Verification items for the finished model (mm, model axes). A direction names the side the tool comes from. Round coordinates to 2 decimals unless told otherwise and drop trailing zeros. Order: outer loops, then holes, each group sorted by start corner. A loop starts at its lowest first (then second) coordinate and runs counter-clockwise, first axis right, second up. Notation, with made-up numbers: M 3.25,6.25 L 21.25,6.25 A24 ccw 21.25,38.25 Z; hole C 56,26 d4. An arc over 180 degrees is marked long. Return JSON: item names as keys, results as strings. Group by question number.
from build123d import *

# Parameters (mm, degrees)
F1_DEPTH     = 10
F2_SIZE      = 5
F3_T1_DEPTH  = 22.73867608
F3_T3_DEPTH  = 22.73867608
F3_T5_DEPTH  = 22.762654105
F3_T7_DEPTH  = 22.8342533194
F3_T9_DEPTH  = 22.7705922303
F3_T11_DEPTH = 22.7699440814
F0_W         = 1.5501256289
F0_H         = 2
F4_DEPTH     = 9.9305


# Not quite as in the source:
# - a fillet or chamfer that OpenCascade refuses, or shapes differently, is made with other operations: its cross-section is extruded or revolved along the edge and cut away or added


with BuildPart() as f1:
    # F0 (on Front) → F1 (new body, symmetric)
    with BuildSketch(Plane.XZ):
        Polygon((-9.3917044375, -16.4117172223), (9.5171118155, -16.3393132389), (19.091183747, 0.0319395585), (9.3917044375, 16.4117172223), (-9.5171118155, 16.3393132389), (-18.908816253, -0.0724039835), align=None)
        with BuildLine():
            ThreePointArc((9.9498743711, -1), (-10, 0), (9.9498743711, 1))
            Line((9.9498743711, 1), (11.5, 1))
            Line((11.5, 1), (11.5, -1))
            Line((11.5, -1), (9.9498743711, -1))
        make_face(mode=Mode.SUBTRACT)
    extrude(amount=F1_DEPTH, both=True)

    # F2
    f2_edges = [f1.edges().sort_by_distance(p)[0] for p in [
        (-14.212964, -10, 8.133455),
        (-14.15026, -10, -8.242061),
        (14.241444, -10, 8.221828),
        (0.062704, -10, -16.375515),
        (14.304148, -10, -8.153687),
        (-0.062704, -10, 16.375515),
    ]]
    chamfer(f2_edges, length=F2_SIZE)

    # F3: fillet of radius 4.6368466753 on 6 edges, made by hand

    # F3_s2 → F3_t1 (cut)
    with BuildSketch(Plane(origin=(5.6469256621, 0, 9.8678304624), x_dir=(0, 1, 0), z_dir=(-0.4966802502, 0, -0.8679335972))):
        with BuildLine():
            ThreePointArc((-10, -9.4549905003), (-9.6470410634, -11.2294349014), (-8.6418990521, -12.7337362278))
            Line((-8.6418990521, -12.7337362278), (-10, -11.3756352799))
            Line((-10, -11.3756352799), (-10, -9.4549905003))
        make_face()
    extrude(amount=F3_T1_DEPTH, mode=Mode.SUBTRACT)

    # F3_s4 → F3_t3 (cut)
    with BuildSketch(Plane(origin=(-5.7223290296, 0, 9.8242963078), x_dir=(0, 1, 0), z_dir=(0.5033124188, 0, -0.8641045128))):
        with BuildLine():
            ThreePointArc((-8.6418990521, -12.7337362278), (-9.6470410634, -11.2294349014), (-10, -9.4549905003))
            Line((-10, -9.4549905003), (-10, -11.3756352799))
            Line((-10, -11.3756352799), (-8.6418990521, -12.7337362278))
        make_face()
    extrude(amount=F3_T3_DEPTH, mode=Mode.SUBTRACT)

    # F3_s6 → F3_t5 (cut)
    with BuildSketch(Plane(origin=(11.393232541, 0, 0.0436259684), x_dir=(0, 1, 0), z_dir=(-0.999992669, 0, -0.0038290844))):
        with BuildLine():
            ThreePointArc((-10, -9.4549905003), (-9.6470410634, -11.2294349014), (-8.6418990521, -12.7337362278))
            Line((-8.6418990521, -12.7337362278), (-10, -11.3756352799))
            Line((-10, -11.3756352799), (-10, -9.4549905003))
        make_face()
    extrude(amount=F3_T5_DEPTH, mode=Mode.SUBTRACT)

    # F3_s8 → F3_t7 (cut)
    with BuildSketch(Plane(origin=(5.8897484246, 0, -9.9461802651), x_dir=(0, 1, 0), z_dir=(-0.5095280522, 0, 0.8604540453))):
        with BuildLine():
            ThreePointArc((-10, -9.5227156054), (-9.6470410634, -11.2971600064), (-8.6418990521, -12.8014613328))
            Line((-8.6418990521, -12.8014613328), (-10, -11.443360385))
            Line((-10, -11.443360385), (-10, -9.5227156054))
        make_face()
    extrude(amount=F3_T7_DEPTH, mode=Mode.SUBTRACT)

    # F3_s10 → F3_t9 (cut)
    with BuildSketch(Plane(origin=(-5.677308487, 0, -9.7079542659), x_dir=(0, 1, 0), z_dir=(0.5048217704, 0, 0.863223598))):
        with BuildLine():
            ThreePointArc((-8.6418990521, -12.8219374878), (-9.6470410634, -11.3176361614), (-10, -9.5431917603))
            Line((-10, -9.5431917603), (-10, -11.4638365399))
            Line((-10, -11.4638365399), (-8.6418990521, -12.8219374878))
        make_face()
    extrude(amount=F3_T9_DEPTH, mode=Mode.SUBTRACT)

    # F3_s12 → F3_t11 (cut)
    with BuildSketch(Plane(origin=(-11.3692546917, 0, -0.0435341545), x_dir=(0, 1, 0), z_dir=(0.999992669, 0, 0.0038290844))):
        with BuildLine():
            ThreePointArc((-8.6418990521, -12.7337362278), (-9.6470410634, -11.2294349014), (-10, -9.4549905003))
            Line((-10, -9.4549905003), (-10, -11.3756352799))
            Line((-10, -11.3756352799), (-8.6418990521, -12.7337362278))
        make_face()
    extrude(amount=F3_T11_DEPTH, mode=Mode.SUBTRACT)

    # F0 (on Front) → F4 (join)
    with BuildSketch(Plane.XZ):
        with Locations((10.7249371855, 0)):
            Rectangle(F0_W, F0_H)
    extrude(amount=F4_DEPTH)


solid = f1.part
1. Cross-section at A-A (y = 1). Enter the section's corners in (x, z).
2. Cross-section at B-B (y = -3). Enter the section's corners in (x, z), plus the area to 3 significant figures.
3. Cross-section at D-D (x = 16.5). Enter the section's corners in (y, z), plus the area to 3 significant figures.
4. Access from +Z, -Z, +X, -X, +Y, -Y to the whole of each face (thin tool, end or side, straight path). Record for faces 4 (the face through (11, 5, 1)), 5 (the face through (-5, -10, 9)).
5. Go/stop test with flat-tipped pins: pin 1 (2 mm diameter, centred on y = -7, z = 0, fed in from -X); pin 2 (4 mm diameter, centred on x = 13.5, y = 0.5, fed in from -Z); pin 3 (1 mm diameter, centred on y = 7.5, z = -12.5, fed in from -X). Record where each tip stops, or that it passes through.
6. Draft check along X on faces 1 (the face through (11.5, 5, 0)), 2 (the face through (14.237, 2.395, -8.268)), 3 (the face through (-5, -10, -9)). Enter one of: +X half, -X half, draft (parallel to the pull), parting line (faces both ways), or undercut.
7. Thickness scan on line 1 along Z through (x, y) = (-9, -6.75); line 2 along Z through (x, y) = (-3.5, -1); line 3 along X through (y, z) = (-7.75, -1.5). Record the ranges inside material, lowest first. Write a range as from..to.
8. Cross-section at C-C (x = -16). Enter the section's corners in (y, z).
Computed:
{
 "1": {"outline": "M -18.91,-0.07 L -9.39,-16.41 L 9.52,-16.34 L 19.09,0.03 L 9.39,16.41 L -9.52,16.34 Z; hole M 9.95,-1 L 11.5,-1 L 11.5,1 L 9.95,1 A10 ccw long Z"},
 "2": {"outline": "M -18.91,-0.07 L -9.39,-16.41 L 9.52,-16.34 L 19.09,0.03 L 9.39,16.41 L -9.52,16.34 Z; hole M 9.95,-1 L 9.95,1 A10 ccw long Z", "area": "618 mm²"},
 "3": {"outline": "M -7.23,0.02 L -5,-4.4 L 10,-4.4 L 10,4.41 L -5,4.41 Z", "area": "142 mm²"},
 "4": {"face 4": "+Y", "face 5": "+Z, -Z, +X, -X, -Y"},
 "5": {"pin 1": "stops at x = -17.75", "pin 2": "stops at z = -12.95", "pin 3": "stops at x = -11.96"},
 "6": {"face 1": "undercut", "face 2": "+X half", "face 3": "draft"},
 "7": {"line 1": "z = -13.61..-4.36, 4.36..13.72", "line 2": "z = -16.39..-9.37, 9.37..16.36", "line 3": "x = -14.89..-9.89, 9.89..15.01"},
 "8": {"outline": "M -7.52,-0.06 L -5,-5.07 L 10,-5.07 L 10,5.01 L -5,5.01 Z"}
}
